```python
from build123d import *

# Parameters (mm, degrees)
SKETCH2_W       = 7
SKETCH2_H       = 1.2
SLOT_DEPTH      = 0.8
THDSCHPAT_COUNT = 14
THDSCHPAT_PITCH = 0.569230769


with BuildPart() as part:
    # BodySke → Base-Revolve (revolve)
    with BuildSketch(Plane.XY):
        with BuildLine():
            Line((2.6, 1.75), (2.6, 3.5))
            Line((2.6, 3.5), (1.4, 3.5))
            ThreePointArc((1.4, 3.5), (0.410050506, 3.089949494), (0, 2.1))
            Line((0, 2.1), (0, 0))
            Line((0, 0), (10.6, 0))
            Line((10.6, 0), (10.6, 1.75))
            Line((10.6, 1.75), (2.6, 1.75))
        make_face()
    revolve(axis=Axis((-25.4, 0, 0), (1, 0, 0)))

    # Sketch2 → Slot (cut)
    with BuildSketch(Plane(origin=(0, 0, 0), x_dir=(0, 0, -1), z_dir=(1, 0, 0))):
        Rectangle(SKETCH2_W, SKETCH2_H)
    extrude(amount=SLOT_DEPTH, mode=Mode.SUBTRACT)

    # ThdSchSke → ThreadSchematic (revolve, cut)
    with BuildSketch(Plane.XY):
        Polygon((3.2, -1.4145), (2.965080371, -1.75), (2.965080371, -2.1875), (3.434919629, -2.1875), (3.434919629, -1.75), align=None)
    threadschematic = revolve(axis=Axis((-3.175, 0, 0), (1, 0, 0)), mode=Mode.SUBTRACT)

    # ThdSchPat: ThreadSchematic ×14
    with Locations(*[(i * THDSCHPAT_PITCH, 0, 0) for i in range(1, THDSCHPAT_COUNT)]):
        add(threadschematic, mode=Mode.SUBTRACT)


solid = part.part
```
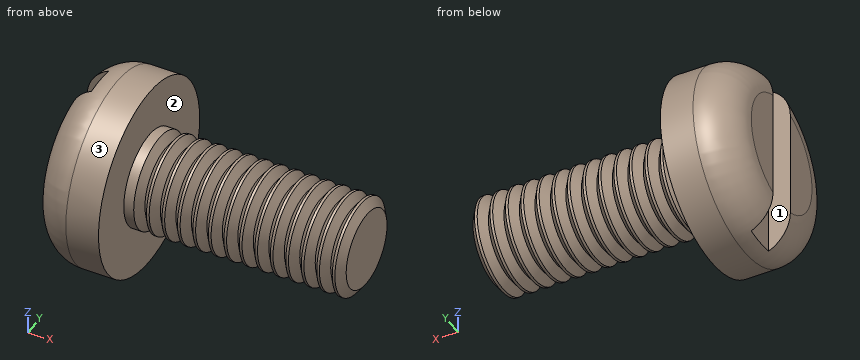
For this review, take the finished solid that the model builds, in its own axes (mm). Face numbers are marked on the shaded views. Coordinates: 2 decimals unless noted, no trailing zeros. Loops run counter-clockwise (first coordinate to the right, second up) from the corner with the lowest first, then second, coordinate; pieces in that order, holes last. Notation, with made-up numbers: (-17.75, 49.25) -> (34.25, 49.25) arc R24 ccw to (34.25, 62.25) -> close; hole circle Ø8 at (26, -25). An arc over 180 degrees is marked (long way). Return JSON: item names as keys, results as strings. Group by question number.
(1) For pin 1 Ø4 at (x, y) = (5, 2) entering from +Z; pin 2 Ø3 at (x, z) = (3.5, 2) entering from +Y; pin 3 Ø3 at (x, z) = (8, -1) entering from +Y, all flat-tipped, find the tip position at first contact; note any pin that passes through.
(2) Consider section B-B, the plane x = 1. Give the boundary of the cut face in (y, z).
(3) Mouldability with a two-part tool opening along Y and no side actions: class the marked faces 1, 2 and 3 as pulls with the +Y half, pulls with the -Y half, needs draft (parallel to the pull), parting line crosses it, or undercut.
(4) To check wall thickness, follow L1, parallel to X at y = 1.75, z = -0.5; L2, parallel to X at y = 0, z = 3.25; L3, parallel to Y at x = 0.75, z = 2.75. State the ranges of each line that lie inside material, in increasing order.
(5) Consider section A-A, the plane x = 2.25. Give the boundary of the cut face in (y, z).
Results below:
{
 "1": {"pin 1": "stops at z = 1.75", "pin 2": "stops at y = 3.41", "pin 3": "stops at y = 1.75"},
 "2": {"outline": "circle Ø6.88 at (0, 0)"},
 "3": {"face 1": "undercut", "face 2": "needs draft", "face 3": "parting line crosses it"},
 "4": {"L1": "x = 0 to 2.6", "L2": "x = 0.8 to 2.6", "L3": "y = -1.9 to -0.6, 0.6 to 1.9"},
 "5": {"outline": "circle Ø7 at (0, 0)"}
}
